Input: part model. Units: mm. Frame: model coordinates. Coordinates: 2 decimals unless noted, no trailing zeros. Loops run counter-clockwise (first coordinate to the right, second up) from the corner with the lowest first, then second, coordinate; pieces in that order, holes last. Notation, with made-up numbers: M -9.75,57 L 11.25,57 A24 ccw 11.25,77 Z; hole C 11,-0.5 d9. An arc over 180 degrees is marked long. Use a Markdown table: item, result. Add a question column.
1. Section A-A on x = 0. Output: boundary loops of the cut face in (y, z), then the cut area to 3 significant figures.
2. Section D-D on z = 0. Output: boundary loops of the cut face in (x, y), then the cut area to 3 significant figures.
3. Section B-B on y = -0.75. Output: boundary loops of the cut face in (x, z).
4. Section C-C on z = -15. Output: boundary loops of the cut face in (x, y).
5. Line query: L1, parallel to Z at x = 25, y = -1.75; L2, parallel to Z at x = 7, y = -1.4 (3 decimals); L3, parallel to X at y = -0.55, z = 10. Output: solid intervals per line, ascending. Write a range as [from, to].
```python
from build123d import *

# Parameters (mm, degrees)
F0_R     = 2.75
F0_R_2   = 12.5
F1_DEPTH = 3


with BuildPart() as f1:
    # F0 (on Front) → F1 (new body)
    with BuildSketch(Plane.XZ):
        with BuildLine():
            Line((45, -25), (15.742295, 12.336131))
            ThreePointArc((15.742295, 12.336131), (0, 20), (-15.742295, 12.336131))
            Line((-15.742295, 12.336131), (-45, -25))
            Line((-45, -25), (-45, -70))
            Line((-45, -70), (45, -70))
            Line((45, -70), (45, -25))
        make_face()
        with Locations((-25, -15)):
            Circle(F0_R, mode=Mode.SUBTRACT)
        with Locations((25, -15)):
            Circle(F0_R, mode=Mode.SUBTRACT)
        Circle(F0_R_2, mode=Mode.SUBTRACT)
    extrude(amount=F1_DEPTH)


solid = f1.part
```
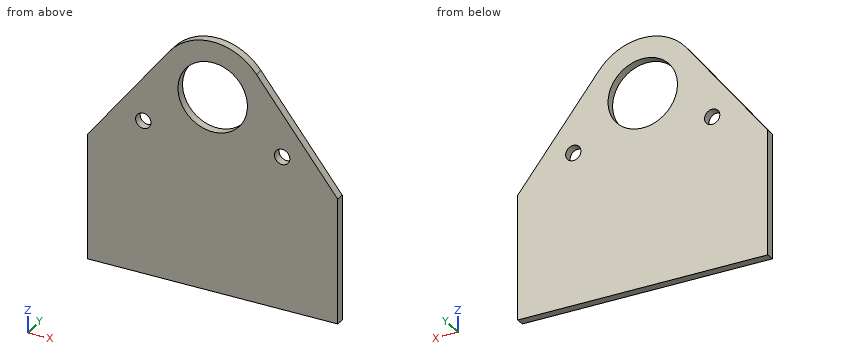
Answers below:
| question | item | result |
|---|---|---|
| 1 | outline | M -3,-70 L 0,-70 L 0,-12.5 L -3,-12.5 Z; M -3,12.5 L 0,12.5 L 0,20 L -3,20 Z |
| 1 | area | 195 mm² |
| 2 | outline | M -25.41,-3 L -12.5,-3 L -12.5,0 L -25.41,0 Z; M 12.5,-3 L 25.41,-3 L 25.41,0 L 12.5,0 Z |
| 2 | area | 77.5 mm² |
| 3 | outline | M -45,-70 L 45,-70 L 45,-25 L 15.74,12.34 A20 ccw -15.74,12.34 L -45,-25 Z; hole C -25,-15 d5.5; hole C 0,0 d25; hole C 25,-15 d5.5 |
| 4 | outline | M -37.16,-3 L -27.75,-3 L -27.75,0 L -37.16,0 Z; M -22.25,-3 L 22.25,-3 L 22.25,0 L -22.25,0 Z; M 27.75,-3 L 37.16,-3 L 37.16,0 L 27.75,0 Z |
| 5 | L1 | z = [-70, -17.75], [-12.25, 0.52] |
| 5 | L2 | z = [-70, -10.356], [10.356, 18.735] |
| 5 | L3 | x = [-17.57, -7.5], [7.5, 17.57] |
